Input: part model. Units: mm. Frame: model coordinates. Give positions to 0.01 mm unless a question says otherwise; leave off trailing zeros. Order: outer loops, then holes, each group sorted by start corner. A loop starts at its lowest first (then second) coordinate and runs counter-clockwise, first axis right, second up. Notation, with made-up numbers: (-21, 31) - (18, 31) arc R11 cw to (18, 37) - close; hole circle Ø8 at (75, 72.25). An arc over 180 degrees is marked (long way). Answer in a Markdown table with one row per item. Add a question column.
1. Ray query, line 1 (Y direction, x = 0.95, z = -52.5); line 2 (Z direction, x = 1.05, y = 262); line 3 (Z direction, x = 0.55, y = 266.5). Return the intervals inside material, ascending. Write a range as [from, to].
2. Section query C-C on z = -48. Return loops of the section in (x, y).
3. Section query A-A on x = 0.55. Return loops of the section in (y, z).
4. Section query B-B on y = 333. Return loops of the section in (x, z), and give its area (3 significant figures).
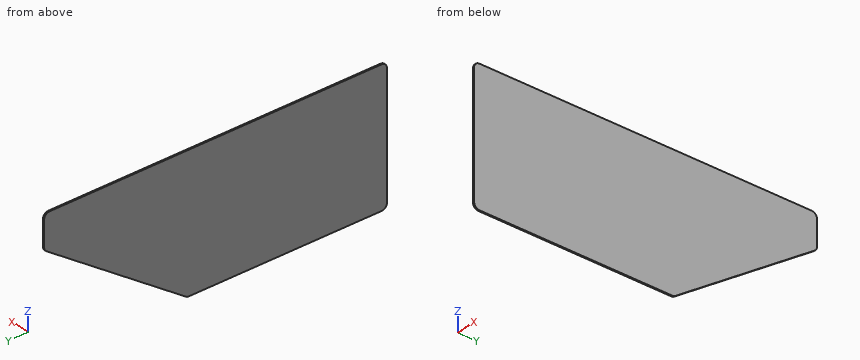
```python
from build123d import *

# Parameters (mm, degrees)
SKETCH1_W           = 1.5875
SKETCH1_H           = 155.8925
BOSS_EXTRUDE1_DEPTH = 400.05
CUT_EXTRUDE1_DEPTH  = 1.5875
FILLET1_R           = 6.35


with BuildPart() as part:
    # Sketch1 → Boss-Extrude1 (new body)
    with BuildSketch(Plane(origin=(0, 0, 0), x_dir=(1, 0, 0), z_dir=(0, 1, 0))):
        with Locations((0.79375, 77.94625)):
            Rectangle(SKETCH1_W, SKETCH1_H)
    extrude(amount=BOSS_EXTRUDE1_DEPTH)

    # Sketch2 → Cut-Extrude1 (cut)
    with BuildSketch(Plane.ZY):
        Polygon((-39.043266439, 400.05), (-155.8925, 233.172), (-155.8925, 400.05), align=None)
    extrude(amount=-CUT_EXTRUDE1_DEPTH, mode=Mode.SUBTRACT)

    # Fillet1
    fillet1_edges = [part.edges().sort_by_distance(p)[0] for p in [
        (0.79375, 400.05, -39.043266439),
        (0.79375, 233.172, -155.8925),
        (0.79375, 400.05, 0),
        (0.79375, 0, -155.8925),
        (0.79375, 0, 0),
    ]]
    fillet(fillet1_edges, radius=FILLET1_R)


solid = part.part
```
Answer:
| question | item | result |
|---|---|---|
| 1 | line 1 | y = [0, 380.83] |
| 1 | line 2 | z = [-135.71, 0] |
| 1 | line 3 | z = [-132.56, 0] |
| 2 | outline | (0, 0) - (1.59, 0) - (1.59, 387.26) - (0, 387.26) - close |
| 3 | outline | (0, -149.54) arc R6.35 ccw to (6.35, -155.89) - (231.17, -155.89) arc R6.35 ccw to (234.81, -154.74) - (397.34, -40.94) arc R6.35 ccw to (400.05, -35.74) - (400.05, -6.35) arc R6.35 ccw to (393.7, 0) - (6.35, 0) arc R6.35 ccw to (0, -6.35) - close |
| 4 | outline | (0, -85.99) - (1.59, -85.99) - (1.59, 0) - (0, 0) - close |
| 4 | area | 137 mm² |
